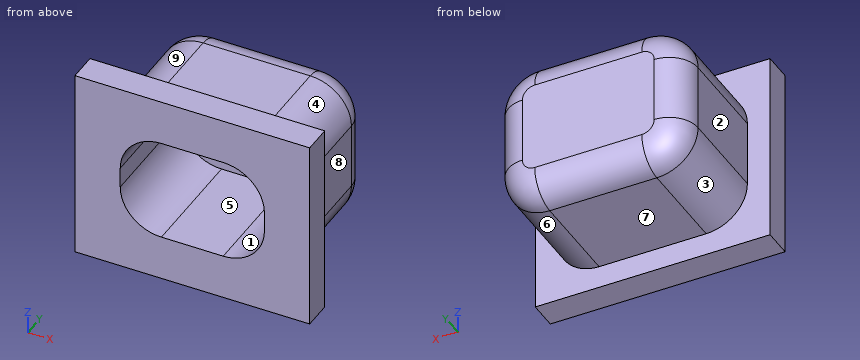
from build123d import *

# Parameters (mm, degrees)
EXTRUDE_332_DEPTH     = 3
SKETCH_2_W            = 5.7
SKETCH_2_H            = 4.7
EXTRUDE_566_DEPTH     = 0.7
CUT_EXTRUDE_806_DEPTH = 2.8
FILLET_1_R            = 0.7


with BuildPart() as part:
    # 草图1 → Extrude 332 (new body)
    with BuildSketch(Plane(origin=(0, 0, 0), x_dir=(1, 0, 0), z_dir=(0, 1, 0))):
        with BuildLine():
            Line((-1.3, -1.8), (1.3, -1.8))
            ThreePointArc((1.3, -1.8), (2.007106781, -1.507106781), (2.3, -0.8))
            Line((2.3, -0.8), (2.3, 0.8))
            ThreePointArc((2.3, 0.8), (2.007106781, 1.507106781), (1.3, 1.8))
            Line((1.3, 1.8), (-1.3, 1.8))
            ThreePointArc((-1.3, 1.8), (-2.007106781, 1.507106781), (-2.3, 0.8))
            Line((-2.3, 0.8), (-2.3, -0.8))
            ThreePointArc((-2.3, -0.8), (-2.007106781, -1.507106781), (-1.3, -1.8))
        make_face()
    extrude(amount=EXTRUDE_332_DEPTH)

    # 草图2 → Extrude 566 (add)
    with BuildSketch(Plane.XZ):
        Rectangle(SKETCH_2_W, SKETCH_2_H)
    extrude(amount=EXTRUDE_566_DEPTH)

    # 草图3 → Cut-Extrude 806 (cut)
    with BuildSketch(Plane.XZ.offset(0.7)):
        with BuildLine():
            Line((-0.75, -1.25), (0.75, -1.25))
            ThreePointArc((0.75, -1.25), (1.457106781, -0.957106781), (1.75, -0.25))
            Line((1.75, -0.25), (1.75, 0.25))
            ThreePointArc((1.75, 0.25), (1.457106781, 0.957106781), (0.75, 1.25))
            Line((0.75, 1.25), (-0.75, 1.25))
            ThreePointArc((-0.75, 1.25), (-1.457106781, 0.957106781), (-1.75, 0.25))
            Line((-1.75, 0.25), (-1.75, -0.25))
            ThreePointArc((-1.75, -0.25), (-1.457106781, -0.957106781), (-0.75, -1.25))
        make_face()
    extrude(amount=-CUT_EXTRUDE_806_DEPTH, mode=Mode.SUBTRACT)

    # 圆角1
    fillet_1_edges = [part.edges().sort_by_distance(p)[0] for p in [
        (2.007106781, 3, -1.507106781),
        (0, 3, -1.8),
        (-2.007106781, 3, -1.507106781),
        (-2.3, 3, 0),
        (-2.007106781, 3, 1.507106781),
        (0, 3, 1.8),
        (2.007106781, 3, 1.507106781),
        (2.3, 3, 0),
    ]]
    fillet(fillet_1_edges, radius=FILLET_1_R)


solid = part.part
Could you check a few things on this model? Use its own coordinates, in mm. Face numbers are marked on the shaded views. A direction names the side the tool comes from. Coordinates: 2 decimals unless noted, no trailing zeros. Order: outer loops, then holes, each group sorted by start corner. A loop starts at its lowest first (then second) coordinate and runs counter-clockwise, first axis right, second up.
Q1. Will these pins go through, and if not, where does the flat tip stop? pin 1 (1.3 mm diameter, centred on y = 1, z = 0.5, fed in from -X); pin 2 (0.7 mm diameter, centred on x = 0.5, y = 1, fed in from +Z); pin 3 (0.5 mm diameter, centred on y = 1, z = 0.5, fed in from +X); pin 4 (1 mm diameter, centred on x = -0.5, z = -1.5, fed in from +Y).
Q2. Suppose I cut it at B-B on x = -0.1. Please give me the cut outline in (y, z), and give its area (3 significant figures).
Q3. Suppose I cut it at C-C on y = 1.3. Please give me the cut outline in (x, z).
Q4. Which directions (+Z, -Z, +X, -X, +Y, -Y) give clear straight access to the entire face, cutting with the end or side of a thin tool? Please do the marked faces 5, 6, 7, 8 and 9.
Q5. Please list where these lines run through material, in increasing order: L1, parallel to Z at x = 0.8, y = -0.05; L2, parallel to X at y = 1.15, z = -0.1; L3, parallel to X at y = -0.2, z = 0.3.
Q6. Suppose I cut it at D-D on z = 1.9. Please give me the cut outline in (x, y).
Q7. Suppose I cut it at A-A on y = -0.35. Please give me the cut outline in (x, z).
Q8. Thinking about a two-plate mould opening in Z: for the marked faces 1, 2, 3 and 4, which applies, released by +Z, released by -Z, zero draft, split by the parting line, or undercut?
Answer:
1. pin 1: stops at x = -2.3
1. pin 2: stops at z = 1.8
1. pin 3: stops at x = 2.3
1. pin 4: stops at y = 3
2. outline: (-0.7, -2.35) - (0, -2.35) - (0, -1.8) - (2.3, -1.8) arc R0.7 ccw to (3, -1.1) - (3, 1.1) arc R0.7 ccw to (2.3, 1.8) - (0, 1.8) - (0, 2.35) - (-0.7, 2.35) - (-0.7, 1.25) - (2.1, 1.25) - (2.1, -1.25) - (-0.7, -1.25) - close
2. area: 6.88 mm2
3. outline: (-2.3, -0.8) arc R1 ccw to (-1.3, -1.8) - (1.3, -1.8) arc R1 ccw to (2.3, -0.8) - (2.3, 0.8) arc R1 ccw to (1.3, 1.8) - (-1.3, 1.8) arc R1 ccw to (-2.3, 0.8) - close; hole (-1.75, -0.25) arc R1 ccw to (-0.75, -1.25) - (0.75, -1.25) arc R1 ccw to (1.75, -0.25) - (1.75, 0.25) arc R1 ccw to (0.75, 1.25) - (-0.75, 1.25) arc R1 ccw to (-1.75, 0.25) - close
4. face 5: -Y
4. face 6: -Z, +X, +Y
4. face 7: -Z, +X, -X, +Y
4. face 8: +Z, -Z, +X, +Y
4. face 9: +Z, -X, +Y
5. L1: z = -2.35 to -1.25, 1.25 to 2.35
5. L2: x = -2.3 to -1.75, 1.75 to 2.3
5. L3: x = -2.85 to -1.75, 1.75 to 2.85
6. outline: (-2.85, -0.7) - (2.85, -0.7) - (2.85, 0) - (-2.85, 0) - close
7. outline: (-2.85, -2.35) - (2.85, -2.35) - (2.85, 2.35) - (-2.85, 2.35) - close; hole (-1.75, -0.25) arc R1 ccw to (-0.75, -1.25) - (0.75, -1.25) arc R1 ccw to (1.75, -0.25) - (1.75, 0.25) arc R1 ccw to (0.75, 1.25) - (-0.75, 1.25) arc R1 ccw to (-1.75, 0.25) - close
8. face 1: undercut
8. face 2: zero draft
8. face 3: released by -Z
8. face 4: released by +Z
